Verification items for the finished model (mm, model axes). Give positions to 0.01 mm unless a question says otherwise; leave off trailing zeros. Loops run counter-clockwise (first coordinate to the right, second up) from the corner with the lowest first, then second, coordinate; pieces in that order, holes last. Notation, with made-up numbers: (27, -30) -> (85, -30) arc R18 ccw to (85, -6) -> close; hole circle Ø9 at (23.25, -28). An arc over 180 degrees is marked (long way). Answer in a Markdown table with one row per item. Add a question column.
Q1. Material ranges on probe 1 along X at (y, z) = (-43, 3); probe 2 along Y at (x, z) = (4, 0.9); probe 3 along X at (y, z) = (-46.5, 1.4), recorded low to high.
Q2. Section check A-A on y = -9. Enter the section's corners in (x, z).
Q3. Section check C-C on y = 22.5. Enter the section's corners in (x, z), and give its area (3 significant figures).
Q4. Gauge pin test, flat ends, axial feed: P1, Ø6.5, axis at x = 0, y = -29, coming from the -Z side; P2, Ø1.5, axis at x = 12, z = 3, coming from the -Y side; P3, Ø1.5, axis at y = 17, z = 3.5, coming from the +X side; P4, Ø1.5, axis at y = 40.5, z = 3, coming from the -X side. Record the tip position at first contact, or that the pin passes through.
Q5. Section check B-B on x = 0. Enter the section's corners in (y, z), and give its area (3 significant figures).
Q6. Section check D-D on z = 1.5. Give the number of separate pieces and of enclosed holes in the cut face, and give its area (3 significant figures).
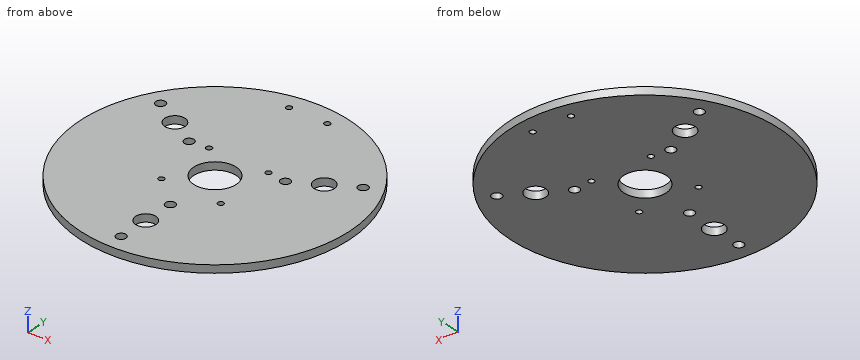
Autodesk Inventor part; units mm, degrees
ref_plane "YZ Plane" through (0, 0, 0) normal (1, 0, 0) x (0, 1, 0)
ref_plane "XZ Plane" through (0, 0, 0) normal (0, 1, 0) x (-1, 0, 0)
ref_plane "XY Plane" through (0, 0, 0) normal (0, 0, 1) x (1, 0, 0)
sketch "Sketch1" plane through (0, 0, 0) normal (0, 0, 1) x (1, 0, 0)
  circle A0 centre (0, 0) radius 70
  circle A1 centre (0, -45) radius 5.25
  circle A2 centre (0, 0) radius 11
  circle A3 centre (10.001, 60.58) radius 1.5
  circle A4 centre (-10.001, 60.58) radius 1.5
  circle A5 centre (15.4998, 15.4998) radius 1.5
  circle A6 centre (0, -29) radius 2.5
  circle A7 centre (0, -61) radius 2.5
  circle A8 centre (52.8275, 30.5) radius 2.5
  circle A9 centre (38.9711, 22.5) radius 5.25
  circle A10 centre (25.1147, 14.5) radius 2.5
  circle A11 centre (-52.8275, 30.5) radius 2.5
  circle A12 centre (-38.9711, 22.5) radius 5.25
  circle A13 centre (-25.1147, 14.5) radius 2.5
  circle A14 centre (0, 0) radius 21.92 construction
  circle A15 centre (-15.4998, 15.4998) radius 1.5
  circle A16 centre (-15.4998, -15.4998) radius 1.5
  circle A17 centre (15.4998, -15.4998) radius 1.5
  dimension "d53" = 43.84
  dimension "D_B" = 140
  dimension "Furos" = 10.5
  dimension "d11" = 22
  dimension "d24" = 3
  dimension "d25" = 3
  dimension "FN" = 3
  dimension "d31" = 5
  dimension "d32" = 5
  dimension "d34" = 16
  dimension "d35" = 16
  dimension "d36" = 10.001
  dimension "d37" = 10.001
  dimension "d38" = 60.58
  dimension "d39" = 60.58
  dimension "d40" = 45
  dimension "d50" = 360
  dimension "d56" = 360
  dimension "d58" = 15.4998
  dimension "d59" = 15.4998
extrude "Extrusion1" add sketch "Sketch1" along normal blind 4
properties part number "test_topo"
Taken from the geometry:
| question | item | result |
|---|---|---|
| 1 | probe 1 | x = -55.24 to -4.85, 4.85 to 55.24 |
| 1 | probe 2 | y = -69.89 to -48.4, -41.6 to -10.25, 10.25 to 69.89 |
| 1 | probe 3 | x = -52.32 to -5.03, 5.03 to 52.32 |
| 2 | outline | (-69.42, 0) -> (-6.32, 0) -> (-6.32, 4) -> (-69.42, 4) -> close; (6.32, 0) -> (69.42, 0) -> (69.42, 4) -> (6.32, 4) -> close |
| 3 | outline | (-66.29, 0) -> (-44.22, 0) -> (-44.22, 4) -> (-66.29, 4) -> close; (-33.72, 0) -> (33.72, 0) -> (33.72, 4) -> (-33.72, 4) -> close; (44.22, 0) -> (66.29, 0) -> (66.29, 4) -> (44.22, 4) -> close |
| 3 | area | 446 mm² |
| 4 | P1 | stops at z = 0 |
| 4 | P2 | stops at y = -69.09 |
| 4 | P3 | stops at x = 68.09 |
| 4 | P4 | stops at x = -57.62 |
| 5 | outline | (-70, 0) -> (-63.5, 0) -> (-63.5, 4) -> (-70, 4) -> close; (-58.5, 0) -> (-50.25, 0) -> (-50.25, 4) -> (-58.5, 4) -> close; (-39.75, 0) -> (-31.5, 0) -> (-31.5, 4) -> (-39.75, 4) -> close; (-26.5, 0) -> (-11, 0) -> (-11, 4) -> (-26.5, 4) -> close; (11, 0) -> (70, 0) -> (70, 4) -> (11, 4) -> close |
| 5 | area | 390 mm² |
| 6 | separate pieces | 1 |
| 6 | enclosed holes | 16 |
| 6 | area | 14,600 mm² |
